Source: CAD feature listing. Evaluate the final solid. Frame: model axes, mm. Face numbers are marked on the shaded views. Give positions to 0.01 mm unless a question says otherwise; leave off trailing zeros. Loops run counter-clockwise (first coordinate to the right, second up) from the corner with the lowest first, then second, coordinate; pieces in that order, holes last. Notation, with made-up numbers: M 45.25,29.25 L 85.25,29.25 A25 ccw 85.25,44.25 Z; hole C -36,-15 d4. An arc over 180 degrees is marked long. Write item = value, one per line.
from build123d import *

# Parameters (mm, degrees)
SKETCH1_R           = 4.5
BOSS_EXTRUDE1_DEPTH = 8
BOSS_EXTRUDE2_START = 6
SKETCH2_R           = 4.5
SKETCH2_R_2         = 2.175
BOSS_EXTRUDE2_DEPTH = 6
BOSS_EXTRUDE3_START = 1.5
SKETCH3_R           = 4.5
BOSS_EXTRUDE3_DEPTH = 1.5
BOSS_EXTRUDE4_START = 13
SKETCH4_R           = 4.5
BOSS_EXTRUDE4_DEPTH = 13


with BuildPart() as part:
    # Sketch1 → Boss-Extrude1 (new body)
    with BuildSketch(Plane(origin=(0, 0, 0), x_dir=(1, 0, 0), z_dir=(0, 1, 0))):
        with Locations(Location((0, 0, 0), (0, 0, 270))):
            Circle(SKETCH1_R)
        with BuildLine():
            ThreePointArc((-0.909869568, -1.991090343), (-0.907761332, -1.974465286), (-0.906473122, -1.957756676))
            ThreePointArc((-0.906473122, -1.957756676), (-1.062514579, -1.653304957), (-1.404275568, -1.63783847))
            ThreePointArc((-1.404275568, -1.63783847), (-1.418939112, -1.645951275), (-1.433186003, -1.654775291))
            ThreePointArc((-1.433186003, -1.654775291), (-1.638194551, -1.758833668), (-1.86090652, -1.815895294))
            ThreePointArc((-1.86090652, -1.815895294), (-1.965014118, -1.702694426), (-2.062246708, -1.58353633))
            ThreePointArc((-2.062246708, -1.58353633), (-1.97407067, -1.371211963), (-1.841895699, -1.183099158))
            ThreePointArc((-1.841895699, -1.183099158), (-1.831133954, -1.170253069), (-1.821016886, -1.15689335))
            ThreePointArc((-1.821016886, -1.15689335), (-1.787688286, -0.816409885), (-2.066834111, -0.618628708))
            ThreePointArc((-2.066834111, -0.618628708), (-2.083555984, -0.617525923), (-2.100311854, -0.617246707))
            ThreePointArc((-2.100311854, -0.617246707), (-2.329034225, -0.593950196), (-2.5472413, -0.521546309))
            ThreePointArc((-2.5472413, -0.521546309), (-2.573621175, -0.370030862), (-2.590996705, -0.217220785))
            ThreePointArc((-2.590996705, -0.217220785), (-2.402027082, -0.086273727), (-2.18913296, 0.00051765))
            ThreePointArc((-2.18913296, 0.00051765), (-2.173134484, 0.00550623), (-2.157400655, 0.01127544))
            ThreePointArc((-2.157400655, 0.01127544), (-1.945283594, 0.279689557), (-2.073187428, 0.596991297))
            ThreePointArc((-2.073187428, 0.596991297), (-2.086658552, 0.606959546), (-2.100603532, 0.616253345))
            ThreePointArc((-2.100603532, 0.616253345), (-2.280421989, 0.759508267), (-2.424844966, 0.938389944))
            ThreePointArc((-2.424844966, 0.938389944), (-2.365121694, 1.080114886), (-2.297123554, 1.218060823))
            ThreePointArc((-2.297123554, 1.218060823), (-2.067356867, 1.226055807), (-1.841335974, 1.183970107))
            ThreePointArc((-1.841335974, 1.183970107), (-1.825180169, 1.179517339), (-1.80882496, 1.175864357))
            ThreePointArc((-1.80882496, 1.175864357), (-1.485265106, 1.28698954), (-1.421318385, 1.623070784))
            ThreePointArc((-1.421318385, 1.623070784), (-1.427261774, 1.638739648), (-1.43396843, 1.654097314))
            ThreePointArc((-1.43396843, 1.654097314), (-1.507791885, 1.871828221), (-1.532577488, 2.10039402))
            ThreePointArc((-1.532577488, 2.10039402), (-1.405712785, 2.18733179), (-1.273929906, 2.266616727))
            ThreePointArc((-1.273929906, 2.266616727), (-1.076315454, 2.149121286), (-0.908927826, 1.991520422))
            ThreePointArc((-0.908927826, 1.991520422), (-0.897744047, 1.979040027), (-0.88596012, 1.96712465))
            ThreePointArc((-0.88596012, 1.96712465), (-0.55368544, 1.885679438), (-0.318190798, 2.133836765))
            ThreePointArc((-0.318190798, 2.133836765), (-0.314719467, 2.15023149), (-0.312058484, 2.166777073))
            ThreePointArc((-0.312058484, 2.166777073), (-0.25644851, 2.389855941), (-0.153727486, 2.595537835))
            ThreePointArc((-0.153727486, 2.595537835), (-0.076897381, 2.598948939), (0, 2.600086305))
            ThreePointArc((0, 2.600086305), (0.076897381, 2.598948939), (0.153727486, 2.595537835))
            ThreePointArc((0.153727486, 2.595537835), (0.25644851, 2.389855941), (0.312058484, 2.166777073))
            ThreePointArc((0.312058484, 2.166777073), (0.314719467, 2.15023149), (0.318190798, 2.133836765))
            ThreePointArc((0.318190798, 2.133836765), (0.55368544, 1.885679438), (0.88596012, 1.96712465))
            ThreePointArc((0.88596012, 1.96712465), (0.897744047, 1.979040027), (0.908927826, 1.991520422))
            ThreePointArc((0.908927826, 1.991520422), (1.076315454, 2.149121286), (1.273929906, 2.266616727))
            ThreePointArc((1.273929906, 2.266616727), (1.405712785, 2.18733179), (1.532577488, 2.10039402))
            ThreePointArc((1.532577488, 2.10039402), (1.507791885, 1.871828221), (1.43396843, 1.654097314))
            ThreePointArc((1.43396843, 1.654097314), (1.427261774, 1.638739648), (1.421318385, 1.623070784))
            ThreePointArc((1.421318385, 1.623070784), (1.485265106, 1.28698954), (1.80882496, 1.175864357))
            ThreePointArc((1.80882496, 1.175864357), (1.825180169, 1.179517339), (1.841335974, 1.183970107))
            ThreePointArc((1.841335974, 1.183970107), (2.067356867, 1.226055807), (2.297123554, 1.218060823))
            ThreePointArc((2.297123554, 1.218060823), (2.365121694, 1.080114886), (2.424844966, 0.938389944))
            ThreePointArc((2.424844966, 0.938389944), (2.280421989, 0.759508267), (2.100603532, 0.616253345))
            ThreePointArc((2.100603532, 0.616253345), (2.086658552, 0.606959546), (2.073187428, 0.596991297))
            ThreePointArc((2.073187428, 0.596991297), (1.945283594, 0.279689557), (2.157400655, 0.01127544))
            ThreePointArc((2.157400655, 0.01127544), (2.173134484, 0.00550623), (2.18913296, 0.00051765))
            ThreePointArc((2.18913296, 0.00051765), (2.402027082, -0.086273727), (2.590996705, -0.217220785))
            ThreePointArc((2.590996705, -0.217220785), (2.573621175, -0.370030862), (2.5472413, -0.521546309))
            ThreePointArc((2.5472413, -0.521546309), (2.329034225, -0.593950196), (2.100311854, -0.617246707))
            ThreePointArc((2.100311854, -0.617246707), (2.083555984, -0.617525923), (2.066834111, -0.618628708))
            ThreePointArc((2.066834111, -0.618628708), (1.787688286, -0.816409885), (1.821016886, -1.15689335))
            ThreePointArc((1.821016886, -1.15689335), (1.831133954, -1.170253069), (1.841895699, -1.183099158))
            ThreePointArc((1.841895699, -1.183099158), (1.97407067, -1.371211963), (2.062246708, -1.58353633))
            ThreePointArc((2.062246708, -1.58353633), (1.965014118, -1.702694426), (1.86090652, -1.815895294))
            ThreePointArc((1.86090652, -1.815895294), (1.638194552, -1.758833667), (1.433186005, -1.65477529))
            ThreePointArc((1.433186005, -1.65477529), (1.418939115, -1.645951274), (1.40427557, -1.637838469))
            ThreePointArc((1.40427557, -1.637838469), (1.06251458, -1.653304956), (0.906473122, -1.957756676))
            ThreePointArc((0.906473122, -1.957756676), (0.907761332, -1.974465287), (0.909869568, -1.991090343))
            ThreePointArc((0.909869568, -1.991090343), (0.919360768, -2.220800089), (0.878747953, -2.447090278))
            ThreePointArc((0.878747953, -2.447090278), (0.732528963, -2.49476454), (0.583747068, -2.533710353))
            ThreePointArc((0.583747068, -2.533710353), (0.427239681, -2.365299878), (0.311033722, -2.166924412))
            ThreePointArc((0.311033722, -2.166924412), (0.303819099, -2.151798727), (0.295869453, -2.13704609))
            ThreePointArc((0.295869453, -2.13704609), (0, -1.965287386), (-0.295869453, -2.13704609))
            ThreePointArc((-0.295869453, -2.13704609), (-0.303819099, -2.151798726), (-0.311033722, -2.166924412))
            ThreePointArc((-0.311033722, -2.166924412), (-0.427239681, -2.365299878), (-0.583747068, -2.533710353))
            ThreePointArc((-0.583747068, -2.533710353), (-0.732528963, -2.49476454), (-0.878747953, -2.447090278))
            ThreePointArc((-0.878747953, -2.447090278), (-0.919360769, -2.220800089), (-0.909869568, -1.991090343))
        make_face(mode=Mode.SUBTRACT)
    extrude(amount=BOSS_EXTRUDE1_DEPTH)

    # Sketch2 → Boss-Extrude2 (add)
    with BuildSketch(Plane.XZ.offset(BOSS_EXTRUDE2_START)):
        with Locations(Location((0, 0, 0), (0, 0, 270))):
            Circle(SKETCH2_R)
        with Locations(Location((0, 0, 0), (0, 0, 98.053222352))):
            Circle(SKETCH2_R_2, mode=Mode.SUBTRACT)
    extrude(amount=-BOSS_EXTRUDE2_DEPTH)

    # Sketch3 → Boss-Extrude3 (add)
    with BuildSketch(Plane.XZ.offset(6).offset(BOSS_EXTRUDE3_START)):
        with Locations(Location((0, 0, 0), (0, 0, 270))):
            Circle(SKETCH3_R)
    extrude(amount=-BOSS_EXTRUDE3_DEPTH)

    # Sketch4 → Boss-Extrude4 (add)
    with BuildSketch(Plane.XZ.offset(7.5).offset(BOSS_EXTRUDE4_START)):
        with Locations(Location((0, 0, 0), (0, 0, 270))):
            Circle(SKETCH4_R)
        with BuildLine():
            Line((-1.747140521, 2.5), (1.747140521, 2.5))
            ThreePointArc((1.747140521, 2.5), (0, -3.05), (-1.747140521, 2.5))
        make_face(mode=Mode.SUBTRACT)
    extrude(amount=-BOSS_EXTRUDE4_DEPTH)


solid = part.part
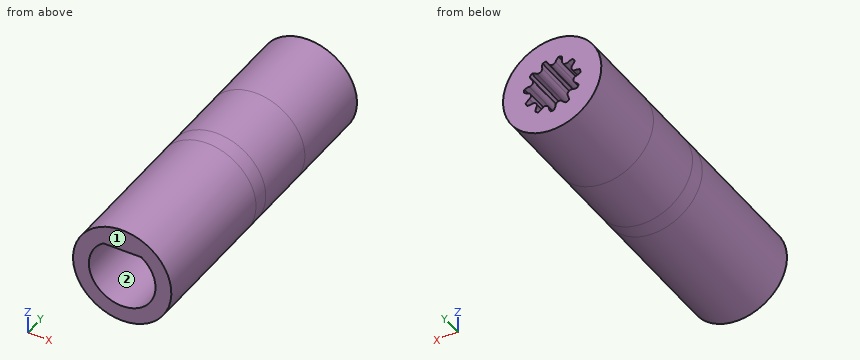
1. Pull-direction query (X, two-part tool) for the marked faces 1 and 2; classes: +X half, -X half, draft (parallel to the pull), parting line (faces both ways), or undercut.
Derived:
face_1 = draft
face_2 = undercut
2. Material intervals for probe 1 along Z at (x, y) = (0, -3.95) (3 decimals); probe 2 along X at (y, z) = (-12.5, 0), sorted ascending. Write a range as from..to.
Derived:
probe_1 = -4.5..-2.175, 2.175..4.5
probe_2 = -4.5..-3.05, 3.05..4.5
3. Cut plane A-A, the plane y = -6.75. Return the cut outline in (x, z), then the cut area to 3 significant figures.
Derived:
outline = C 0,0 d9
area = 63.6 mm²
4. Cut plane C-C, the plane z = 3.25. Return the cut outline in (x, y).
Derived:
outline = M -3.11,-20.5 L 3.11,-20.5 L 3.11,8 L -3.11,8 Z
5. Cut plane B-B, the plane y = -0.75. Return the cut outline in (x, z) (3 decimals).
Derived:
outline = C 0,0 d9; hole C 0,0 d4.35
6. First-contact query: pin 1 Ø1.7 at (x, z) = (-1.5, 0.5) entering from -Y; pin 2 Ø1.5 at (y, z) = (1, 3) entering from +X; pin 3 Ø1.5 at (x, y) = (1, -16) entering from +Z. Flat tips, straight axial feed; report the tip coordinate or a pass-through.
Derived:
pin_1 = -7.5
pin_2 = 3.9
pin_3 = 4.49
